from build123d import *

# Parameters (mm, degrees)
F0_R     = 406.4
F0_R_2   = 203.2
F1_DEPTH = 76.2
F0_R_3   = 152.4
F2_DEPTH = 457.2
F3_DEPTH = 754.38
F4_SIZE  = 25.4
F5_DEPTH = 76.2


with BuildPart() as f1:
    # F0 (on Front) → F1 (new body, symmetric)
    with BuildSketch(Plane.XZ):
        Circle(F0_R)
        Circle(F0_R_2, mode=Mode.SUBTRACT)
    extrude(amount=F1_DEPTH, both=True)

    # F0 (on Front) → F2 (join)
    with BuildSketch(Plane.XZ):
        Circle(F0_R_2)
        Circle(F0_R_3, mode=Mode.SUBTRACT)
    extrude(amount=F2_DEPTH)

    # F0 (on Front) → F3 (cut)
    with BuildSketch(Plane.XZ):
        Circle(F0_R_3)
    extrude(amount=-F3_DEPTH, mode=Mode.SUBTRACT)

    # F4
    f4_edges = [f1.edges().sort_by_distance(p)[0] for p in [
        (-203.2, -457.2, 0),
    ]]
    chamfer(f4_edges, length=F4_SIZE)

    # F5 (add): a face of the model
    f5_faces = [f1.faces().sort_by_distance(p)[0] for p in [
        (-197.4526360825, 0, 0),
    ]]
    extrude(f5_faces, amount=F5_DEPTH)


solid = f1.part
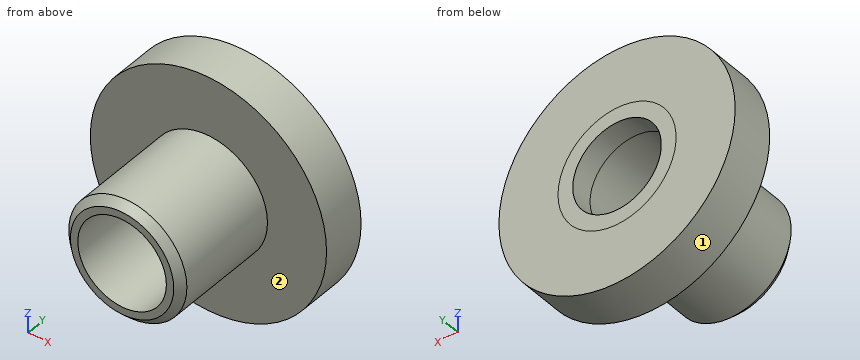
Design review of the part built by this model. Coordinates are the model's own, in mm. Face numbers are marked on the shaded views. A direction names the side the tool comes from. Coordinates: 2 decimals unless noted, no trailing zeros. Write each loop counter-clockwise with the first axis right and the second up, starting at its lowest first coordinate (ties: lowest second). Pieces come first, ordered by that corner, then holes. Notation, with made-up numbers: (-38.5, 64.25) - (18.5, 64.25) arc R25 cw to (18.5, 86.25) - close; hole circle Ø10 at (66, 43). An arc over 180 degrees is marked (long way). Use one line per item in the form item = value.
Q1. Consider section A-A (x = 0). Write out the cut boundary in (y, z), plus the area to 3 significant figures.
Taken from the geometry:
outline = (-457.2, -177.8) - (-431.8, -203.2) - (-76.2, -203.2) - (-76.2, -406.4) - (76.2, -406.4) - (76.2, -152.4) - (-457.2, -152.4) - close; (-457.2, 152.4) - (76.2, 152.4) - (76.2, 406.4) - (-76.2, 406.4) - (-76.2, 203.2) - (-431.8, 203.2) - (-457.2, 177.8) - close
area = 115,000 mm^2
Q2. Consider section D-D (x = 264.5). Write out the cut boundary in (y, z).
Taken from the geometry:
outline = (-76.2, -308.55) - (76.2, -308.55) - (76.2, 308.55) - (-76.2, 308.55) - close
Q3. Consider section B-B (z = 0). Write out the cut boundary in (x, y).
Taken from the geometry:
outline = (-406.4, -76.2) - (-203.2, -76.2) - (-203.2, -431.8) - (-177.8, -457.2) - (-152.4, -457.2) - (-152.4, 76.2) - (-406.4, 76.2) - close; (152.4, -457.2) - (177.8, -457.2) - (203.2, -431.8) - (203.2, -76.2) - (406.4, -76.2) - (406.4, 76.2) - (152.4, 76.2) - close
Q4. Insertion check: pin 1 Ø3 at (y, z) = (-67.5, 166) entering from +X; pin 2 Ø2 at (y, z) = (-6, 127) entering from +X; pin 3 Ø4 at (y, z) = (-359, 1.5) entering from +X. Each pin has a flat end and moves straight along its axis. Give the tip position at first contact, or say it passes through.
Taken from the geometry:
pin_1 = 371.62
pin_2 = 386.37
pin_3 = 203.2
Q5. Machinability: for the marked faces 1 and 2, which of the approach directions +Z, -Z, +X, -X, +Y, -Y give a long, thin tool a straight path to every point of the face, cutting with its end or side? Answer none if there is none.
Taken from the geometry:
face_1 = +Y, -Y
face_2 = -Y
Q6. For probe 1 along Z at (x, y) = (0, 39); probe 2 along Z at (x, y) = (0, -332.5); probe 3 along Y at (x, z) = (-67, -275), list the stretches that pass through material, from the lowest coordinate up.
Taken from the geometry:
probe_1 = -406.4 to -152.4, 152.4 to 406.4
probe_2 = -203.2 to -152.4, 152.4 to 203.2
probe_3 = -76.2 to 76.2
Q7. Consider section C-C (y = -245). Write out the cut boundary in (x, z), plus the area to 3 significant figures.
Taken from the geometry:
outline = circle Ø406.4 at (0, 0); hole circle Ø304.8 at (0, 0)
area = 56,800 mm^2
